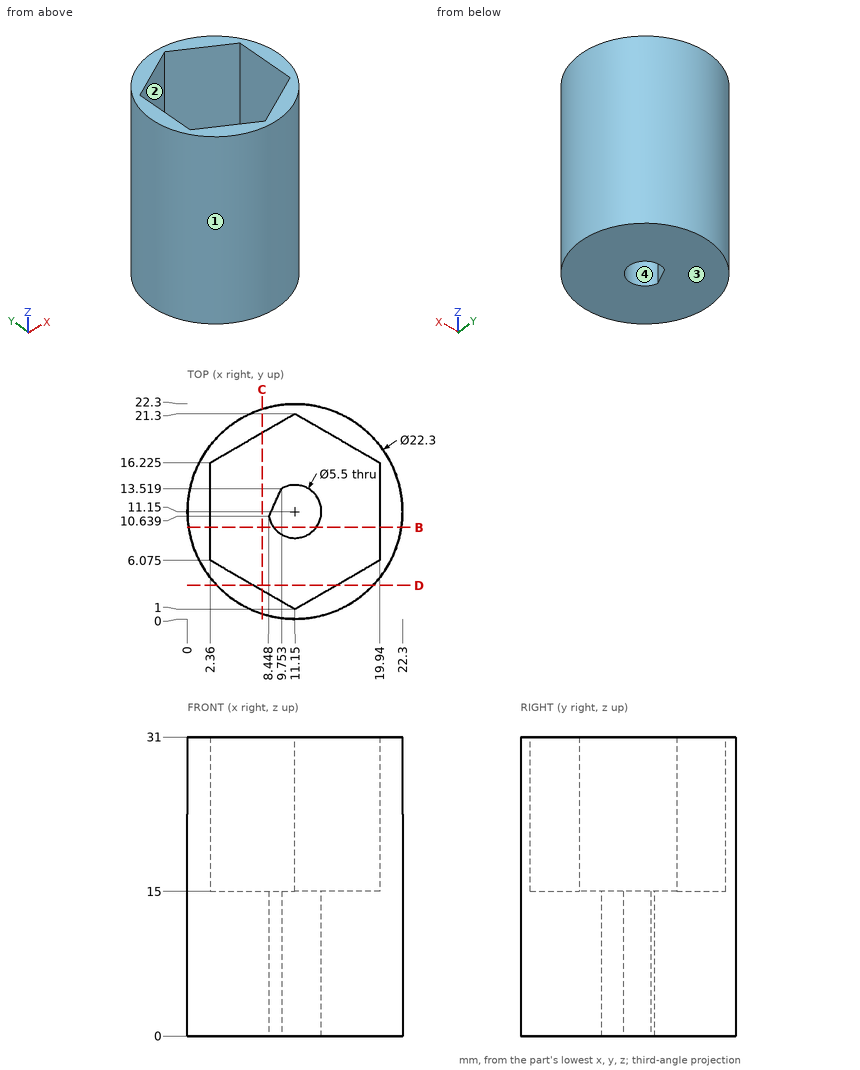
Print and shaded views of the part. All mm, measured from the part's lowest x, y and z. Coordinates: 2 decimals unless noted, no trailing zeros. Order: outer loops, then holes, each group sorted by start corner. A loop starts at its lowest first (then second) coordinate and runs counter-clockwise, first axis right, second up. Notation, with made-up numbers: (18.5, -15) -> (66.5, -15) arc R15 cw to (66.5, 2) -> close; hole circle Ø4 at (-27, 77). An arc over 180 degrees is marked (long way). Answer as a JSON object with one key per item and string values. Group by question number.
1) Cut at D-D, the plane y = 3.5. Write the cut outline in (x, z).
2) Pull direction X, two halves, no side cores. Call the marked faces 1, 2, 3 and 4: +X half, -X half, draft (parallel to the pull), parting line (faces both ways), or undercut.
3) Drill centre lines: L1, parallel to Y at x = 11.25, z = 14; L2, parallel to Z at x = 3, y = 10.25; L3, parallel to X at y = 11.25, z = 21. Where is each one in solid material? Low to high.
4) Flat gauge pins, fed straight in: pin 1 (3 mm diameter, centred on y = 13.5, z = 23, fed in from +X); pin 2 (10 mm diameter, centred on x = 8.5, y = 10, fed in from +Z); pin 3 (2 mm diameter, centred on y = 18, z = 16.5, fed in from -X). Where does each tip first touch, or does it go through?
5) Cut at C-C, the plane x = 7.75. Write the cut outline in (y, z).
6) Cut at B-B, the plane y = 9.5. Write the cut outline in (x, z).
Check values:
{
 "1": {"outline": "(3.04, 0) -> (19.26, 0) -> (19.26, 31) -> (15.48, 31) -> (15.48, 15) -> (6.82, 15) -> (6.82, 31) -> (3.04, 31) -> close"},
 "2": {"face 1": "parting line", "face 2": "undercut", "face 3": "draft", "face 4": "undercut"},
 "3": {"L1": "y = 0 to 8.4, 13.9 to 22.3", "L2": "z = 0 to 15", "L3": "x = 0 to 2.36, 19.94 to 22.3"},
 "4": {"pin 1": "stops at x = 22.27", "pin 2": "stops at z = 15", "pin 3": "stops at x = 1.66"},
 "5": {"outline": "(0.53, 0) -> (21.77, 0) -> (21.77, 31) -> (19.34, 31) -> (19.34, 15) -> (2.96, 15) -> (2.96, 31) -> (0.53, 31) -> close"},
 "6": {"outline": "(0.12, 0) -> (8.95, 0) -> (8.95, 15) -> (2.36, 15) -> (2.36, 31) -> (0.12, 31) -> close; (13.35, 0) -> (22.18, 0) -> (22.18, 31) -> (19.94, 31) -> (19.94, 15) -> (13.35, 15) -> close"}
}
